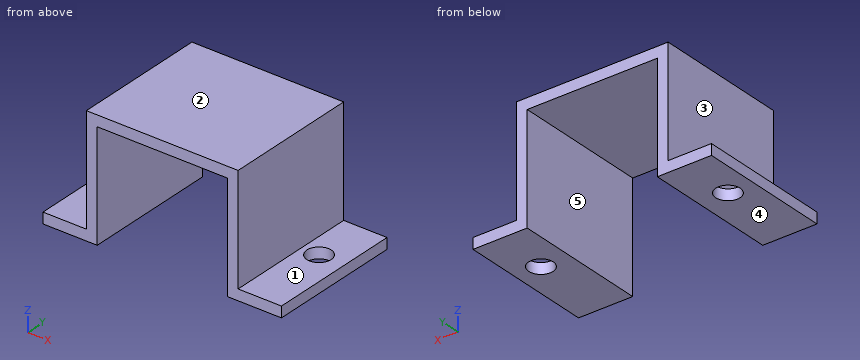
```python
from build123d import *

# Parameters (mm, degrees)
SKETCH2_W           = 14
SKETCH2_H           = 12.5
BOSS_EXTRUDE1_DEPTH = 11
SKETCH3_W           = 12
SKETCH3_H           = 10
CUT_EXTRUDE1_DEPTH  = 12.5
SKETCH4_W           = 1
SKETCH4_H           = 12.5
BOSS_EXTRUDE2_DEPTH = 4
SKETCH5_W           = 1
SKETCH5_H           = 12.5
BOSS_EXTRUDE3_DEPTH = 4
SKETCH6_R           = 1.125
CUT_EXTRUDE2_DEPTH  = 1


with BuildPart() as part:
    # Sketch2 → Boss-Extrude1 (new body)
    with BuildSketch(Plane.XY):
        with Locations((-3.028513908, 0.880933534)):
            Rectangle(SKETCH2_W, SKETCH2_H)
    extrude(amount=BOSS_EXTRUDE1_DEPTH)

    # Sketch3 → Cut-Extrude1 (cut)
    with BuildSketch(Plane(origin=(0, -5.369066466, 0), x_dir=(-1, 0, 0), z_dir=(0, -1, 0))):
        with Locations((3.028513908, -5)):
            Rectangle(SKETCH3_W, SKETCH3_H)
    extrude(amount=-CUT_EXTRUDE1_DEPTH, mode=Mode.SUBTRACT)

    # Sketch4 → Boss-Extrude2 (add)
    with BuildSketch(Plane(origin=(3.971486092, 0, 0), x_dir=(0, 0, -1), z_dir=(1, 0, 0))):
        with Locations((-0.5, 0.880933534)):
            Rectangle(SKETCH4_W, SKETCH4_H)
    extrude(amount=BOSS_EXTRUDE2_DEPTH)

    # Sketch5 → Boss-Extrude3 (add)
    with BuildSketch(Plane.ZY.offset(10.028513908)):
        with Locations((0.5, 0.880933534)):
            Rectangle(SKETCH5_W, SKETCH5_H)
    extrude(amount=BOSS_EXTRUDE3_DEPTH)

    # Sketch6 → Cut-Extrude2 (cut)
    with BuildSketch(Plane.XY.offset(1)):
        with Locations((-11.653513908, 2.130933534)):
            Circle(SKETCH6_R)
        with Locations((5.596486092, 2.130933534)):
            Circle(SKETCH6_R)
    extrude(amount=-CUT_EXTRUDE2_DEPTH, mode=Mode.SUBTRACT)


solid = part.part
```
Source: CAD feature listing. Evaluate the final solid. Frame: model axes, mm. Face numbers are marked on the shaded views. A direction names the side the tool comes from. Give positions to 0.01 mm unless a question says otherwise; leave off trailing zeros. Loops run counter-clockwise (first coordinate to the right, second up) from the corner with the lowest first, then second, coordinate; pieces in that order, holes last. Notation, with made-up numbers: (54, -13) -> (91, -13) arc R32 ccw to (91, 20) -> close; hole circle Ø11 at (44.25, 1.25). An arc over 180 degrees is marked (long way). Use a Markdown table: item, result. Add a question column.
(1) First-contact query: pin 1 Ø3 at (x, y) = (-11, 3) entering from +Z; pin 2 Ø2 at (y, z) = (0, 8) entering from -X; pin 3 Ø6 at (x, z) = (-1.5, 4.5) entering from +Y; pin 4 Ø3 at (y, z) = (-1.5, 5.5) entering from +X. Flat tips, straight axial feed; report the tip coordinate or a pass-through.
(2) Ray query, line 1 (X direction, y = 1, z = 3); line 2 (Z direction, x = 6.25, y = -1.5); line 3 (Z direction, x = -2.75, y = 5.5). Return the intervals inside material, ascending.
(3) Access query for the marked faces 1, 2, 3, 4 and 5. Directions: +Z, -Z, +X, -X, +Y, -Y. A direction counts if a zero-diameter tool reaches every point of the face in a straight line with its end or side. Return the directions, or none.
(4) Section query A-A (z = 9.75). Output: boundary loops of the cut face in (x, y), then the cut area to 3 significant figures.
(5) Section query C-C (x = -12.25). Output: boundary loops of the cut face in (y, z), then the cut area to 3 significant figures.
(6) Section query D-D (y = 2.5). Output: boundary loops of the cut face in (x, z), then the cut area to 3 significant figures.
(7) Section query B-B (y = -4.25). Output: boundary loops of the cut face in (x, z), then the cut area to 3 significant figures.
Checked values:
| question | item | result |
|---|---|---|
| 1 | pin 1 | z = 11 |
| 1 | pin 2 | x = -10.03 |
| 1 | pin 3 | through |
| 1 | pin 4 | x = 3.97 |
| 2 | line 1 | -10.03 to -9.03, 2.97 to 3.97 |
| 2 | line 2 | 0 to 1 |
| 2 | line 3 | 10 to 11 |
| 3 | face 1 | +Z, +X, +Y, -Y |
| 3 | face 2 | +Z, +X, -X, +Y, -Y |
| 3 | face 3 | +Z, -X, +Y, -Y |
| 3 | face 4 | -Z, +X, -X, +Y, -Y |
| 3 | face 5 | -Z, +Y, -Y |
| 4 | outline | (-10.03, -5.37) -> (-9.03, -5.37) -> (-9.03, 7.13) -> (-10.03, 7.13) -> close; (2.97, -5.37) -> (3.97, -5.37) -> (3.97, 7.13) -> (2.97, 7.13) -> close |
| 4 | area | 25.0 mm^2 |
| 5 | outline | (-5.37, 0) -> (1.18, 0) -> (1.18, 1) -> (-5.37, 1) -> close; (3.08, 0) -> (7.13, 0) -> (7.13, 1) -> (3.08, 1) -> close |
| 5 | area | 10.6 mm^2 |
| 6 | outline | (-14.03, 0) -> (-12.72, 0) -> (-12.72, 1) -> (-14.03, 1) -> close; (-10.59, 0) -> (-9.03, 0) -> (-9.03, 10) -> (2.97, 10) -> (2.97, 0) -> (4.53, 0) -> (4.53, 1) -> (3.97, 1) -> (3.97, 11) -> (-10.03, 11) -> (-10.03, 1) -> (-10.59, 1) -> close; (6.66, 0) -> (7.97, 0) -> (7.97, 1) -> (6.66, 1) -> close |
| 6 | area | 37.7 mm^2 |
| 7 | outline | (-14.03, 0) -> (-9.03, 0) -> (-9.03, 10) -> (2.97, 10) -> (2.97, 0) -> (7.97, 0) -> (7.97, 1) -> (3.97, 1) -> (3.97, 11) -> (-10.03, 11) -> (-10.03, 1) -> (-14.03, 1) -> close |
| 7 | area | 42.0 mm^2 |
